Geometry check sheet. Reference: the model listing, model coordinates, mm. Coordinates: 2 decimals unless noted, no trailing zeros. Order: outer loops, then holes, each group sorted by start corner. A loop starts at its lowest first (then second) coordinate and runs counter-clockwise, first axis right, second up. Notation, with made-up numbers: (40.25, 43) - (77.25, 43) arc R24 ccw to (77.25, 70) - close; hole circle Ø7 at (19, 82). An arc over 180 degrees is marked (long way). Put each result on its own line as item: value.
from build123d import *

# Parameters (mm, degrees)
F_18_0_1695_DIAMETER_HOLE1_D     = 4.3053
F_18_0_1695_DIAMETER_HOLE1_DEPTH = 38.1
F_18_0_1695_DIAMETER_HOLE1_TIP   = 1.293442612
CUT_EXTRUDE1_DEPTH               = 28


with BuildPart() as part:
    # Sketch2 → Revolve1 (revolve)
    with BuildSketch(Plane.XY, mode=Mode.PRIVATE) as revolve1_sk:
        with BuildLine():
            Line((50, 0), (62.5, 0))
            Line((62.5, 0), (62.5, 7.982495649))
            Line((62.5, 7.982495649), (52.5, 7.982495649))
            ThreePointArc((52.5, 7.982495649), (51.285053929, 8.09980714), (50.114998295, 8.447407131))
            Line((50.114998295, 8.447407131), (23.792498295, 19.114911482))
            ThreePointArc((23.792498295, 19.114911482), (20.911227085, 21.451920296), (19.8275, 25))
            Line((19.8275, 25), (16.8275, 25))
            Line((16.8275, 25), (16.8275, 22))
            ThreePointArc((16.8275, 22), (17.911227085, 18.451920296), (20.792498295, 16.114911482))
            Line((20.792498295, 16.114911482), (46.035001705, 5.885088518))
            ThreePointArc((46.035001705, 5.885088518), (48.916272915, 3.548079704), (50, 0))
        make_face()
    revolve(revolve1_sk.sketch.rotate(Axis((0, 0, 0), (0, 1, 0)), 90), axis=Axis((0, 0, 0), (0, 1, 0)))

    # #18 (0.1695) Diameter Hole1
    with Locations(Plane(origin=(0, 0, 0), x_dir=(-1, 0, 0), z_dir=(0, -1, 0))):
        with Locations((0, 56.25), (0, -56.25), (-56.25, 0), (56.25, 0)):
            Hole(F_18_0_1695_DIAMETER_HOLE1_D / 2, depth=F_18_0_1695_DIAMETER_HOLE1_DEPTH)
            with Locations((0, 0, -(F_18_0_1695_DIAMETER_HOLE1_DEPTH + F_18_0_1695_DIAMETER_HOLE1_TIP / 2))):  # 118° drill point
                Cone(0, F_18_0_1695_DIAMETER_HOLE1_D / 2, F_18_0_1695_DIAMETER_HOLE1_TIP, mode=Mode.SUBTRACT)

    # Sketch5 → Cut-Extrude1 (cut)
    with BuildSketch(Plane(origin=(0, 7.982495649, 0), x_dir=(1, 0, 0), z_dir=(0, 1, 0))):
        with BuildLine():
            Line((-56.597565166, 7.921), (-59.13485528, 7.921))
            ThreePointArc((-59.13485528, 7.921), (-61.28824505, 7.07913898), (-62.299678972, 5))
            ThreePointArc((-62.299678972, 5), (-44.194173824, 44.194173824), (-5, 62.299678972))
            ThreePointArc((-5, 62.299678972), (-7.07913898, 61.28824505), (-7.921, 59.13485528))
            Line((-7.921, 59.13485528), (-7.921, 56.597565166))
            ThreePointArc((-7.921, 56.597565166), (-8.644467885, 54.57998881), (-10.485166883, 53.48187801))
            ThreePointArc((-10.485166883, 53.48187801), (-38.537319575, 38.537319575), (-53.48187801, 10.485166883))
            ThreePointArc((-53.48187801, 10.485166883), (-54.57998881, 8.644467885), (-56.597565166, 7.921))
        make_face()
        with BuildLine():
            Line((7.921, 56.597565166), (7.921, 59.13485528))
            ThreePointArc((7.921, 59.13485528), (7.07913898, 61.28824505), (5, 62.299678972))
            ThreePointArc((5, 62.299678972), (44.194173824, 44.194173824), (62.299678972, 5))
            ThreePointArc((62.299678972, 5), (61.28824505, 7.07913898), (59.13485528, 7.921))
            Line((59.13485528, 7.921), (56.597565166, 7.921))
            ThreePointArc((56.597565166, 7.921), (54.57998881, 8.644467885), (53.48187801, 10.485166883))
            ThreePointArc((53.48187801, 10.485166883), (38.537319575, 38.537319575), (10.485166883, 53.48187801))
            ThreePointArc((10.485166883, 53.48187801), (8.644467885, 54.57998881), (7.921, 56.597565166))
        make_face()
        with BuildLine():
            Line((56.597565166, -7.921), (59.13485528, -7.921))
            ThreePointArc((59.13485528, -7.921), (61.28824505, -7.07913898), (62.299678972, -5))
            ThreePointArc((62.299678972, -5), (44.194173824, -44.194173824), (5, -62.299678972))
            ThreePointArc((5, -62.299678972), (7.07913898, -61.28824505), (7.921, -59.13485528))
            Line((7.921, -59.13485528), (7.921, -56.597565166))
            ThreePointArc((7.921, -56.597565166), (8.644467885, -54.57998881), (10.485166883, -53.48187801))
            ThreePointArc((10.485166883, -53.48187801), (38.537319575, -38.537319575), (53.48187801, -10.485166883))
            ThreePointArc((53.48187801, -10.485166883), (54.57998881, -8.644467885), (56.597565166, -7.921))
        make_face()
        with BuildLine():
            Line((-7.921, -56.597565166), (-7.921, -59.13485528))
            ThreePointArc((-7.921, -59.13485528), (-7.07913898, -61.28824505), (-5, -62.299678972))
            ThreePointArc((-5, -62.299678972), (-44.194173824, -44.194173824), (-62.299678972, -5))
            ThreePointArc((-62.299678972, -5), (-61.28824505, -7.07913898), (-59.13485528, -7.921))
            Line((-59.13485528, -7.921), (-56.597565166, -7.921))
            ThreePointArc((-56.597565166, -7.921), (-54.57998881, -8.644467885), (-53.48187801, -10.485166883))
            ThreePointArc((-53.48187801, -10.485166883), (-38.537319575, -38.537319575), (-10.485166883, -53.48187801))
            ThreePointArc((-10.485166883, -53.48187801), (-8.644467885, -54.57998881), (-7.921, -56.597565166))
        make_face()
    extrude(amount=-CUT_EXTRUDE1_DEPTH, mode=Mode.SUBTRACT)


solid = part.part
Q1. Section check C-C on y = 14.5. Record the boundary of the cut face in (x, z).
Answer block:
outline: circle Ø70.36 at (0, 0); hole circle Ø49.55 at (0, 0)
Q2. Draft check along Z on faces 1 (the cylindrical face through (-7.06, 4.05, -61.31)), 2 (the cylindrical face through (-8.66, 4.05, 54.56)), 3 (the cylindrical face through (-0.47, 4.05, 58.35)). Enter one of: pulls with the +Z half, pulls with the -Z half, needs draft (parallel to the pull), parting line crosses it, or undercut.
Answer block:
face 1: pulls with the -Z half
face 2: pulls with the +Z half
face 3: undercut
Q3. Thickness scan on L1, parallel to Z at x = -56.25, y = 2.5; L2, parallel to X at y = 2.75, z = -5. Record the ranges inside material, lowest first. Write a range as [from, to].
Answer block:
L1: z = [-7.94, -2.15], [2.15, 7.94]
L2: x = [-62.3, -49.12], [49.12, 62.3]
Q4. Depth check by flat-ended pin: pin 1 Ø3 at (x, y) = (-16.5, 9) entering from -Z; pin 2 Ø3 at (x, y) = (-57.5, 6) entering from +Z; pin 3 Ø3 at (x, y) = (58.5, 3.5) entering from -Z. Enter the tip coordinate at first touch or a pass-through.
Answer block:
pin 1: stops at z = -52.28
pin 2: stops at z = 7.98
pin 3: stops at z = -7.92
Q5. Section check A-A on z = 0. State how many separate pieces and enclosed holes the cut face has, then the cut area to 3 significant figures.
Answer block:
separate pieces: 4
enclosed holes: 0
area: 440 mm^2
